```python
from build123d import *

# Parameters (mm, degrees)
ESBO_O1_W                = 175
ESBO_O1_H                = 172.5
RESSALTO_EXTRUS_O1_DEPTH = 10
ESBO_O5_W                = 30
ESBO_O5_H                = 6
RESSALTO_EXTRUS_O5_DEPTH = 10
ESBO_O6_W                = 6
ESBO_O6_H                = 30
RESSALTO_EXTRUS_O6_DEPTH = 10
ESBO_O7_W                = 30
ESBO_O7_H                = 6
RESSALTO_EXTRUS_O7_DEPTH = 10
ESBO_O9_W                = 6.2
ESBO_O9_H                = 172.5
CORTE_EXTRUS_O2_DEPTH    = 5
ESBO_O10_R               = 1.5
CORTE_EXTRUS_O3_DEPTH    = 8
ESBO_O11_R               = 1.5
CORTE_EXTRUS_O4_DEPTH    = 8
CORTE_EXTRUS_O5_DEPTH    = 11


with BuildPart() as part:
    # Esboço1 → Ressalto-extrusão1 (new body)
    with BuildSketch(Plane.XY):
        Rectangle(ESBO_O1_W, ESBO_O1_H)
    extrude(amount=RESSALTO_EXTRUS_O1_DEPTH)

    # Esboço5 → Ressalto-extrusão5 (add)
    with BuildSketch(Plane(origin=(0, 86.25, 0), x_dir=(1, 0, 0), z_dir=(0, 1, 0))):
        with Locations((-37.5, -5)):
            Rectangle(ESBO_O5_W, ESBO_O5_H)
        with Locations((37.5, -5)):
            Rectangle(ESBO_O5_W, ESBO_O5_H)
    extrude(amount=RESSALTO_EXTRUS_O5_DEPTH)

    # Esboço6 → Ressalto-extrusão6 (add)
    with BuildSketch(Plane.ZY.offset(87.5)):
        with Locations((5, 36.25)):
            Rectangle(ESBO_O6_W, ESBO_O6_H)
        with Locations((5, -36.25)):
            Rectangle(ESBO_O6_W, ESBO_O6_H)
    extrude(amount=RESSALTO_EXTRUS_O6_DEPTH)

    # Esboço7 → Ressalto-extrusão7 (add)
    with BuildSketch(Plane.XZ.offset(86.25)):
        with Locations((-37.5, 5)):
            Rectangle(ESBO_O7_W, ESBO_O7_H)
        with Locations((37.5, 5)):
            Rectangle(ESBO_O7_W, ESBO_O7_H)
    extrude(amount=RESSALTO_EXTRUS_O7_DEPTH)

    # Esboço9 → Corte-extrusão2 (cut)
    with BuildSketch(Plane.XY.offset(10)):
        with Locations((79.4, 0)):
            Rectangle(ESBO_O9_W, ESBO_O9_H)
    extrude(amount=-CORTE_EXTRUS_O2_DEPTH, mode=Mode.SUBTRACT)

    # Esboço10 → Corte-extrusão3 (cut)
    with BuildSketch(Plane.ZY.offset(87.5)):
        with Locations((5, -71.25)):
            Circle(ESBO_O10_R)
    extrude(amount=-CORTE_EXTRUS_O3_DEPTH, mode=Mode.SUBTRACT)

    # Esboço11 → Corte-extrusão4 (cut)
    with BuildSketch(Plane.XZ.offset(86.25)):
        with Locations((65, 5)):
            Circle(ESBO_O11_R)
    extrude(amount=-CORTE_EXTRUS_O4_DEPTH, mode=Mode.SUBTRACT)

    # Esboço12 → Corte-extrusão5 (cut, through all)
    with BuildSketch(Plane(origin=(0, 0, 0), x_dir=(-1, 0, 0), z_dir=(0, 0, -1))):
        with BuildLine():
            Line((-3.85, 7.31931366), (-3.85, 0.18068634))
            ThreePointArc((-3.85, 0.18068634), (1.917028951, -1.137484015), (5.25, 3.75))
            ThreePointArc((5.25, 3.75), (1.917028951, 8.637484015), (-3.85, 7.31931366))
        make_face()
    extrude(amount=-CORTE_EXTRUS_O5_DEPTH, mode=Mode.SUBTRACT)


solid = part.part
```
The listing builds one solid part. Answer for the finished solid, in the listing's coordinates (mm). A direction names the side the tool comes from. Coordinates: 2 decimals unless noted, no trailing zeros. Write each loop counter-clockwise with the first axis right and the second up, starting at its lowest first coordinate (ties: lowest second). Pieces come first, ordered by that corner, then holes. Notation, with made-up numbers: M -17,53 L 38,53 A7 cw 38,60 Z; hole C 46.5,-14 d2. An arc over 180 degrees is marked long. Use a Markdown table: item, result. Add a question column.
1. Which of the six approach directions +Z, -Z, +X, -X, +Y, -Y give full straight-line access (tool end or side, diameter ignored) to faces 1 (the flat face through (-38, 91, 8)), 2 (the flat face through (37, -91, 2)), 3 (the flat face through (-92, 36, 8)), 4 (the flat face through (-22.5, 91, 5)), 5 (the flat face through (-52.5, 91, 5))?
2. Given P1, Ø5, axis at x = -94.5, y = -35, coming from the -Z side; P2, Ø3, axis at y = -90.5, z = 4.5, coming from the +X side; P3, Ø1.8, axis at x = -90, z = 6, coming from the -Y side, each flat-ended and moving along its own axis, determine where each tip first touches the part or whether it passes through.
3. Section C-C (x = -33) is taken. Give the vertices of the cut face in (y, z).
4. Straight lines are drawn through the part: line 1 along Z through (x, y) = (-83, -71.25); line 2 along X through (y, z) = (-66, 8.75); line 3 along Y through (x, z) = (5.5, 4.75). For each, find the intervals that lie inside material, in ascending order. Write a range as [from, to].
5. For a pull along X with two mould halves and no side action, classify faces 6 (the flat face through (52.5, 91, 5)), 7 (the flat face through (22.5, 91, 5)), 8 (the flat face through (-7, 1, 10)) as +X half, -X half, draft (parallel to the pull), parting line (faces both ways), or undercut.
6. Section B-B (x = -84) is taken. Give the vertices of the cut face in (y, z).
7. Section A-A (y = -46) is taken. Give the vertices of the cut face in (x, z), plus the area to 3 significant figures.
8. Section D-D (y = -14.5) is taken. Give the vertices of the cut face in (x, z), plus the area to 3 significant figures.
Data:
| question | item | result |
|---|---|---|
| 1 | face 1 | +Z, +X, -X, +Y |
| 1 | face 2 | -Z, +X, -X, -Y |
| 1 | face 3 | +Z, -X, +Y, -Y |
| 1 | face 4 | +Z, -Z, +Y |
| 1 | face 5 | +Z, -Z, -X, +Y |
| 2 | P1 | stops at z = 2 |
| 2 | P2 | stops at x = 52.5 |
| 2 | P3 | stops at y = -51.25 |
| 3 | outline | M -96.25,2 L -86.25,2 L -86.25,0 L 86.25,0 L 86.25,2 L 96.25,2 L 96.25,8 L 86.25,8 L 86.25,10 L -86.25,10 L -86.25,8 L -96.25,8 Z |
| 4 | line 1 | z = [0, 3.5], [6.5, 10] |
| 4 | line 2 | x = [-87.5, 76.3], [82.5, 87.5] |
| 4 | line 3 | y = [-86.25, 86.25] |
| 5 | face 6 | +X half |
| 5 | face 7 | undercut |
| 5 | face 8 | draft |
| 6 | outline | M -86.25,0 L 86.25,0 L 86.25,10 L -86.25,10 Z; hole C -71.25,5 d3 |
| 7 | outline | M -97.5,2 L -87.5,2 L -87.5,0 L 87.5,0 L 87.5,10 L 82.5,10 L 82.5,5 L 76.3,5 L 76.3,10 L -87.5,10 L -87.5,8 L -97.5,8 Z |
| 7 | area | 1,780 mm2 |
| 8 | outline | M -87.5,0 L 87.5,0 L 87.5,10 L 82.5,10 L 82.5,5 L 76.3,5 L 76.3,10 L -87.5,10 Z |
| 8 | area | 1,720 mm2 |
